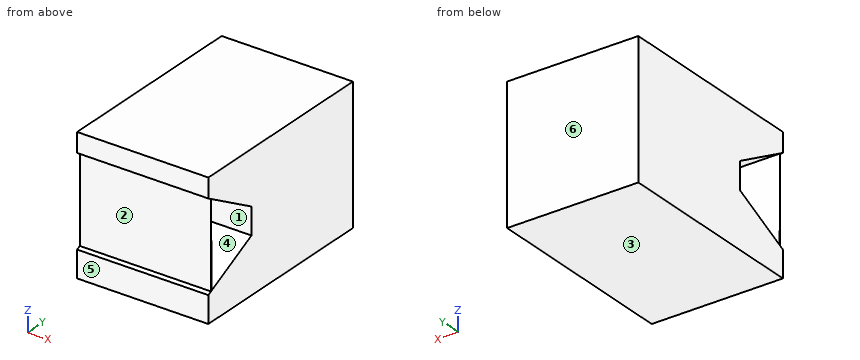
```python
from build123d import *

# Parameters (mm, degrees)
F0_W     = 76.149322
F0_H     = 97.219742
F1_DEPTH = 58
F2_W     = 76.149322
F2_H     = 116
F3_DEPTH = 18.7
F5_DEPTH = 123.1
F7_DEPTH = 89.5


with BuildPart() as f1:
    # F0 (on Front) → F1 (new body, symmetric)
    with BuildSketch(Plane.XZ):
        Rectangle(F0_W, F0_H)
    extrude(amount=F1_DEPTH, both=True)

    # F2 (on face) → F3 (cut)
    with BuildSketch(Plane.XY.offset(48.609871)):
        Rectangle(F2_W, F2_H)
    extrude(amount=-F3_DEPTH, mode=Mode.SUBTRACT)

    # F4 (on Right) → F5 (cut, symmetric)
    with BuildSketch(Plane.YZ):
        Polygon((-23.388904, -0.990585), (-55.867601, 17.457999), (-55.406615, -31.883165), (-23.388904, -16.519183), align=None)
    extrude(amount=F5_DEPTH, both=True, mode=Mode.SUBTRACT)

    # F6 (on Right) → F7 (cut, symmetric)
    with BuildSketch(Plane.YZ):
        Polygon((-55.870809, 17.301733), (-55.870809, 17.458142), (-58.005538, 18.668221), (-58.056336, -33.160523), (-55.870809, -32.10915), align=None)
    extrude(amount=F7_DEPTH, both=True, mode=Mode.SUBTRACT)


solid = f1.part
```
Check sheet for the modelled part. Datum: model origin and axes. Units: mm. Face numbers are marked on the shaded views. A direction names the side the tool comes from. Round coordinates to 2 decimals unless told otherwise and drop trailing zeros. Order: outer loops, then holes, each group sorted by start corner. A loop starts at its lowest first (then second) coordinate and runs counter-clockwise, first axis right, second up. Notation, with made-up numbers: (42, -3.5) -> (49, -3.5) arc R23 cw to (49, 24.5) -> close; hole circle Ø1 at (26.5, 35.25). An arc over 180 degrees is marked (long way). One line per item, written item: value. Start each with the question number.
Q1. Cross-section at B-B (x = -31). Record the boundary of the cut face in (y, z).
Q2. Set-up check for the marked faces 1, 2 and 3: record each of +Z, -Z, +X, -X, +Y, -Y from which the full face is reachable in a straight line by a thin tool's end or side.
Q3. Thickness scan on line 1 (Y direction, x = -15.5, z = -11.5); line 2 (Y direction, x = 1.5, z = -4); line 3 (Z direction, x = -33, y = -44). Record the ranges inside material, lowest first.
Q4. Gauge pin test, flat end, axial feed: pin 1 Ø12.5 at (x, z) = (-12, -6.5) entering from -Y. Record the tip position at first contact, or that the pin passes through.
Q5. Mould release check, pull along Y, two halves, no side actions. Record for the marked faces 4, 5 and 6: pulls with the +Y half, pulls with the -Y half, needs draft (parallel to the pull), parting line crosses it, or undercut.
Q6. Cross-section at A-A (y = -26.5). Record the boundary of the cut face in (x, z), and give its area (3 significant figures).
Completed:
1. outline: (-58, -48.61) -> (58, -48.61) -> (58, 29.91) -> (-58, 29.91) -> (-58, 18.67) -> (-55.87, 17.46) -> (-55.87, -32.11) -> (-58, -33.13) -> close; hole (-55.87, 17.46) -> (-55.41, -31.88) -> (-23.39, -16.52) -> (-23.39, -0.99) -> close
2. face 1: +X, -X
2. face 2: +X, -X, -Y
2. face 3: -Z, +X, -X, +Y, -Y
3. line 1: y = -55.87 to -55.6, -23.39 to 58
3. line 2: y = -55.87 to -55.67, -23.39 to 58
3. line 3: z = -48.61 to -26.41, 10.72 to 29.91
4. pin 1: stops at y = -55.87
5. face 4: undercut
5. face 5: pulls with the -Y half
5. face 6: pulls with the +Y half
6. outline: (-38.07, -48.61) -> (38.07, -48.61) -> (38.07, -18.01) -> (-38.07, -18.01) -> close; (-38.07, 0.78) -> (38.07, 0.78) -> (38.07, 29.91) -> (-38.07, 29.91) -> close
6. area: 4,550 mm²
